Source: CAD feature listing. Evaluate the final solid. Frame: model axes, mm. A direction names the side the tool comes from. Give positions to 0.01 mm unless a question says otherwise; leave off trailing zeros. Loops run counter-clockwise (first coordinate to the right, second up) from the corner with the lowest first, then second, coordinate; pieces in that order, holes last.
Autodesk Inventor part; units mm, degrees
ref_plane "YZ Plane" through (0, 0, 0) normal (1, 0, 0) x (0, 1, 0)
ref_plane "XZ Plane" through (0, 0, 0) normal (0, 1, 0) x (-1, 0, 0)
ref_plane "XY Plane" through (0, 0, 0) normal (0, 0, 1) x (1, 0, 0)
sketch "草图1" plane through (0, 0, 0) normal (0, 0, 1) x (1, 0, 0)
  line L0 (-50, -50) -> (50, -50)
  line L1 (50, -50) -> (50, 50)
  line L2 (50, 50) -> (-50, 50)
  line L3 (-50, 50) -> (-50, -50)
  line L4 (-50, -50) -> (50, 50) construction
  line L5 (50, -50) -> (-50, 50) construction
  point P0 (0, 0)
  dimension "d0" = 100
  dimension "d1" = 100
extrude "拉伸1" add sketch "草图1" along normal blind 6
sketch "草图2" plane through (0, 0, 6) normal (0, 0, 1) x (1, 0, 0)
  line L0 (-25, -25) -> (25, -25)
  line L1 (25, -25) -> (25, 25)
  line L2 (25, 25) -> (-25, 25)
  line L3 (-25, 25) -> (-25, -25)
  line L4 (-25, -25) -> (25, 25) construction
  line L5 (25, -25) -> (-25, 25) construction
  point P0 (0, 0)
  dimension "d4" = 50
  dimension "d5" = 50
extrude "拉伸2" add sketch "草图2" along normal blind 5
sketch "草图3" plane through (0, 0, 11) normal (0, 0, 1) x (1, 0, 0)
  line L0 (-17.5, -17.5) -> (17.5, -17.5)
  line L1 (17.5, -17.5) -> (17.5, 17.5)
  line L2 (17.5, 17.5) -> (-17.5, 17.5)
  line L3 (-17.5, 17.5) -> (-17.5, -17.5)
  line L4 (-17.5, -17.5) -> (17.5, 17.5) construction
  line L5 (17.5, -17.5) -> (-17.5, 17.5) construction
  point P0 (0, 0)
  dimension "d8" = 35
  dimension "d9" = 35
extrude "拉伸3" cut sketch "草图3" against normal through all
sketch "草图4" plane through (0, 0, 11) normal (0, 0, 1) x (1, 0, 0)
  line L0 (-21, -21) -> (21, -21)
  line L1 (21, -21) -> (21, 21)
  line L2 (21, 21) -> (-21, 21)
  line L3 (-21, 21) -> (-21, -21)
  line L4 (-21, -21) -> (21, 21) construction
  line L5 (21, -21) -> (-21, 21) construction
  circle A0 centre (21, 21) radius 2.15
  circle A1 centre (-21, 21) radius 2.15
  circle A2 centre (21, -21) radius 2.15
  circle A3 centre (-21, -21) radius 2.15
  point P0 (0, 0)
  dimension "d12" = 42
  dimension "d13" = 42
  dimension "d14" = 4.3
  dimension "d15" = 4.3
  dimension "d16" = 4.3
  dimension "d17" = 4.3
extrude "拉伸4" cut sketch "草图4" against normal through all contours L3 A3 L0 | L0 A3 L3 | A2 L1 L0 | L0 L1 A2 | A1 L2 L3 | L3 L2 A1 | A0 L2 L1 | L1 L2 A0
sketch "草图5" plane through (0, 0, 0) normal (0, 0, -1) x (-1, 0, 0)
  line L0 (15, 22.5) -> (-15, 22.5)
  line L1 (-15, -17.5) -> (-15, -57.5)
  line L2 (-15, -57.5) -> (15, -57.5)
  line L3 (15, -57.5) -> (15, -17.5)
  line L4 (17.5, -17.5) -> (-17.5, -17.5)
  line L5 (15, 22.5) -> (-15, -57.5) construction
  line L6 (-15, 22.5) -> (15, -57.5) construction
  line L7 (-15, -17.5) -> (15, -17.5)
  line L8 (12.5, -12.5) -> (-12.5, -12.5)
  line L9 (-12.5, -12.5) -> (-12.5, 12.5)
  line L10 (-12.5, 12.5) -> (12.5, 12.5)
  line L11 (12.5, 12.5) -> (12.5, -12.5)
  line L12 (12.5, -12.5) -> (-12.5, 12.5) construction
  line L13 (-12.5, -12.5) -> (12.5, 12.5) construction
  line L14 (17.5, -17.5) -> (-17.5, -17.5)
  line L15 (-17.5, -17.5) -> (-17.5, 17.5)
  line L16 (-17.5, 17.5) -> (17.5, 17.5)
  line L17 (17.5, 17.5) -> (17.5, -17.5)
  line L18 (17.5, -17.5) -> (-17.5, 17.5) construction
  line L19 (-17.5, -17.5) -> (17.5, 17.5) construction
  point P0 (0, 0)
  point P1 (0, -17.5)
  dimension "d20" = 30
  dimension "d21" = 80
  dimension "d22" = 30
  dimension "d23" = 40
  dimension "d31" = 25
  dimension "d32" = 25
sketch "草图6" plane through (-50, -50, 0) normal (0, -1, 0) x (1, 0, 0)
  line L0 (0, 0) -> (0, 6)
  line L1 (100, 0) -> (0, 0)
  line L2 (0, 0) -> (0, 6)
  line L3 (0, 6) -> (100, 6)
  line L4 (100, 6) -> (100, 0)
  point P0 (50, 0)
extrude "拉伸5" add sketch "草图6" along normal blind 15
sketch "草图7" plane through (0, 0, 0) normal (0, 0, -1) x (-1, 0, 0)
  point P0 (0, 0)
extrude "拉伸6" cut sketch "草图5" against normal blind 3 contours L4 L3 L2 L1
sketch "草图8" plane through (0, 0, 0) normal (0, 0, -1) x (-1, 0, 0)
  line L0 (15, -57.5) -> (-15, -57.5)
  line L1 (-9.993, -57.5) -> (10.007, -57.5)
  line L2 (10.007, -57.5) -> (10.007, -69.9689)
  line L3 (10.007, -69.9689) -> (-9.993, -69.9689)
  line L4 (-9.993, -69.9689) -> (-9.993, -57.5)
  line L5 (10.007, -69.9689) -> (0.007, -69.9689)
  point P0 (0, 0)
  dimension "d28" = 20
extrude "拉伸7" cut sketch "草图8" against normal blind 3
sketch "草图9" plane through (0, 0, 11) normal (0, 0, 1) x (1, 0, 0)
  line L0 (17.5, 17.5) -> (17.5, -17.5)
  line L1 (-17.5, -17.5) -> (17.5, -17.5)
  line L2 (17.5, -17.5) -> (17.5, 17.5)
  line L3 (17.5, 17.5) -> (-17.5, 17.5)
  line L4 (-17.5, 17.5) -> (-17.5, -17.5)
  line L5 (-17.5, -17.5) -> (17.5, 17.5) construction
  line L6 (17.5, -17.5) -> (-17.5, 17.5) construction
  line L7 (-12.5, -12.5) -> (12.5, -12.5)
  line L8 (12.5, -12.5) -> (12.5, 12.5)
  line L9 (12.5, 12.5) -> (-12.5, 12.5)
  line L10 (-12.5, 12.5) -> (-12.5, -12.5)
  line L11 (-12.5, -12.5) -> (12.5, 12.5) construction
  line L12 (12.5, -12.5) -> (-12.5, 12.5) construction
  point P0 (0, 0)
  dimension "d33" = 25
  dimension "d34" = 25
extrude "拉伸8" add sketch "草图9" against normal blind 11
sketch "草图10" plane through (0, 0, 0) normal (0, 0, -1) x (-1, 0, 0)
  line L0 (-15, -57.5) -> (-15, -17.5)
  line L1 (-15, -17.5) -> (15, -17.5)
  line L2 (15, -17.5) -> (15, -12.5)
  line L3 (15, -12.5) -> (-15, -12.5)
  line L4 (-15, -12.5) -> (-15, -17.5)
  point P0 (0, 0)
  dimension "d37" = 5
extrude "拉伸9" cut sketch "草图10" against normal blind 3
sketch "草图11" plane through (0, 0, 0) normal (0, 0, -1) x (-1, 0, 0)
  line L0 (-50, -65) -> (-50, 50)
  line L1 (-50, -65) -> (-34.1728, -65)
  line L2 (-34.1728, -65) -> (-34.1728, -62)
  line L3 (-34.1728, -62) -> (-50, -62)
  line L4 (-50, -62) -> (-50, -65)
  line L5 (50, 50) -> (50, -65)
  line L6 (-50, -65) -> (50, -65)
  line L7 (50, -65) -> (50, -62)
  line L8 (50, -62) -> (-50, -62)
  line L9 (-50, -62) -> (-50, -65)
  point P0 (0, 0)
  dimension "d40" = 3
extrude "拉伸10" cut sketch "草图11" against normal blind 11
properties part number "11"
1) Cut plane D-D (y = -21). Return loops of the section in (x, z).
Checks:
outline: (-50, 0) - (-23.15, 0) - (-23.15, 11) - (-25, 11) - (-25, 6) - (-50, 6) - close; (-18.85, 0) - (-15, 0) - (-15, 3) - (15, 3) - (15, 0) - (18.85, 0) - (18.85, 11) - (-18.85, 11) - close; (23.15, 0) - (50, 0) - (50, 6) - (25, 6) - (25, 11) - (23.15, 11) - close
2) Cut plane C-C (z = 9.25). Return loops of the section in (x, y).
Checks:
outline: (-25, -25) - (25, -25) - (25, 25) - (-25, 25) - close; hole circle Ø4.3 at (-21, -21); hole circle Ø4.3 at (-21, 21); hole (-12.5, -12.5) - (12.5, -12.5) - (12.5, 12.5) - (-12.5, 12.5) - close; hole circle Ø4.3 at (21, -21); hole circle Ø4.3 at (21, 21)
3) Cut plane A-A (x = -0.5). Return loops of the section in (y, z), and give its area (4 significant figures).
Checks:
outline: (-62, 3) - (-12.5, 3) - (-12.5, 11) - (-25, 11) - (-25, 6) - (-62, 6) - close; (12.5, 0) - (50, 0) - (50, 6) - (25, 6) - (25, 11) - (12.5, 11) - close
area: 498.5 mm2
4) Pull-direction query (X, two-part tool) for faces 1 (the flat face through (13, -57.5, 1)), 2 (the flat face through (25, 0, 8)), 3 (the flat face through (-25, 0, 8)), 4 (the flat face through (0, 25, 8)); classes: released by +X, released by -X, zero draft, split by the parting line, or undercut.
Checks:
face 1: undercut
face 2: released by +X
face 3: released by -X
face 4: zero draft
5) Ray query, probe 1 along X at (y, z) = (-21, 8.5); probe 2 along Y at (x, z) = (-21, 5.25); probe 3 along X at (y, z) = (21, 4.5). Return the intervals inside material, ascending.
Checks:
probe 1: x = -25 to -23.15, -18.85 to 18.85, 23.15 to 25
probe 2: y = -62 to -23.15, -18.85 to 18.85, 23.15 to 50
probe 3: x = -50 to -23.15, -18.85 to 18.85, 23.15 to 50
6) Cut plane B-B (x = -21). Return loops of the section in (y, z).
Checks:
outline: (-62, 0) - (-23.15, 0) - (-23.15, 11) - (-25, 11) - (-25, 6) - (-62, 6) - close; (-18.85, 0) - (18.85, 0) - (18.85, 11) - (-18.85, 11) - close; (23.15, 0) - (50, 0) - (50, 6) - (25, 6) - (25, 11) - (23.15, 11) - close
7) Reachability of faces 5 (the flat face through (-10.007, -60, 1)), 6 (the flat face through (-1, -30, 6)), 7 (the flat face through (-1, 20, 0)), 8 (the flat face through (-15, -35, 1)) from +Z, -Z, +X, -X, +Y, -Y: full face, straight path, thin tool, end or side. Return the list, or none.
Checks:
face 5: -Z, -Y
face 6: +Z
face 7: -Z, +X, -X, +Y, -Y
face 8: -Z
8) Contact query for flat-ended pins moving along their axis: P1, Ø10, axis at x = -30, y = -39, coming from the +Z side; P2, Ø1.5, axis at y = 7, z = 9.5, coming from the +X side; P3, Ø5, axis at x = 21, y = -21, coming from the -Z side; P4, Ø3.5, axis at x = -21, y = -21, coming from the -Z side. Output: stop coordinate, or through.
Checks:
P1: stops at z = 6
P2: stops at x = 25
P3: stops at z = 0
P4: passes through
